Read the model definition and answer for the solid it produces. Units are mm, in the model's axes. A direction names the side the tool comes from. Coordinates: 2 decimals unless noted, no trailing zeros. Write each loop counter-clockwise with the first axis right and the second up, starting at its lowest first coordinate (ties: lowest second). Pieces come first, ordered by that corner, then holes.
from build123d import *

# Parameters (mm, degrees)
ESQUISSE1_R             = 20
BOSS_EXTRU_1_DEPTH      = 2
ESQUISSE2_R             = 3.025
BOSS_EXTRU_2_DEPTH      = 4
ESQUISSE4_R             = 10
BOSS_EXTRU_3_DEPTH      = 0.5
ENL_V_MAT_EXTRU_1_DEPTH = 6
ESQUISSE5_R             = 4.025
BOSS_EXTRU_4_DEPTH      = 1


with BuildPart() as part:
    # Esquisse1 → Boss.-Extru.1 (new body)
    with BuildSketch(Plane(origin=(0, 0, 0), x_dir=(1, 0, 0), z_dir=(0, 1, 0))):
        Circle(ESQUISSE1_R)
    extrude(amount=BOSS_EXTRU_1_DEPTH)

    # Esquisse2 → Boss.-Extru.2 (add)
    with BuildSketch(Plane(origin=(0, 2, 0), x_dir=(1, 0, 0), z_dir=(0, 1, 0))):
        with Locations((0, 16)):
            Circle(ESQUISSE2_R)
        with Locations((16, 0)):
            Circle(ESQUISSE2_R)
        with Locations((0, -16)):
            Circle(ESQUISSE2_R)
        with Locations((-16, 0)):
            Circle(ESQUISSE2_R)
    extrude(amount=BOSS_EXTRU_2_DEPTH)

    # Esquisse4 → Boss.-Extru.3 (add)
    with BuildSketch(Plane(origin=(0, 2, 0), x_dir=(1, 0, 0), z_dir=(0, 1, 0))):
        Circle(ESQUISSE4_R)
    extrude(amount=BOSS_EXTRU_3_DEPTH)

    # Esquisse3 → Enlèv. mat.-Extru.1 (cut)
    with BuildSketch(Plane(origin=(0, 2.5, 0), x_dir=(1, 0, 0), z_dir=(0, 1, 0))):
        Polygon((4.5, -7.794228634), (9, 0), (4.5, 7.794228634), (-4.5, 7.794228634), (-9, 0), (-4.5, -7.794228634), align=None)
    extrude(amount=-ENL_V_MAT_EXTRU_1_DEPTH, mode=Mode.SUBTRACT)

    # Esquisse5 → Boss.-Extru.4 (add)
    with BuildSketch(Plane(origin=(0, 2, 0), x_dir=(1, 0, 0), z_dir=(0, 1, 0))):
        with Locations((16, 0)):
            Circle(ESQUISSE5_R)
        with Locations((0, 16)):
            Circle(ESQUISSE5_R)
        with Locations((0, -16)):
            Circle(ESQUISSE5_R)
        with Locations((-16, 0)):
            Circle(ESQUISSE5_R)
    extrude(amount=BOSS_EXTRU_4_DEPTH)


solid = part.part
Item 1: The part is cut by section B-B (z = 6). Give the vertices of the cut face in (x, y).
Item 2: For faces 1 (the flat face through (-6.781, 1.268, 3.843)), 2 (the cylindrical face through (2.164, 2.493, -19.394)), 3 (the flat face through (16, 6, 0)), determine the directions among +Z, -Z, +X, -X, +Y, -Y from which every point of the face is accessible in a straight line to the end or side of a thin tool.
Item 3: Given pin 1 (1 mm diameter, centred on y = 3.5, z = 8, fed in from +X); pin 2 (3 mm diameter, centred on y = 3, z = 14.5, fed in from -X); pin 3 (1.5 mm diameter, centred on x = 8.5, y = 2, fed in from +Z); pin 4 (16 mm diameter, centred on x = 1, z = 1.5, fed in from +Y), each flat-ended and moving along its own axis, determine where each tip first touches the part or whether it passes through.
Item 4: Find the intervals of material crossed by probe 1 along Z at (x, y) = (0, 3.2) (3 decimals); probe 2 along Y at (x, z) = (-5.5, -6.5); probe 3 along X at (y, z) = (0.45, 0), in increasing order.
Item 5: The part is cut by section D-D (z = 16). Give the vertices of the cut face in (x, y) (3 decimals), and give its area (3 significant figures).
Item 6: The part is cut by section A-A (x = 0). Give the vertices of the cut face in (y, z) (3 decimals), and give its area (3 significant figures).
Item 7: The part is cut by section C-C (x = -16). Give the vertices of the cut face in (y, z) (3 decimals), and give its area (3 significant figures).
Answer:
1. outline: (-19.08, 0) - (-5.54, 0) - (-5.54, 2.5) - (-8, 2.5) - (-8, 2) - (-19.08, 2) - close; (5.54, 0) - (19.08, 0) - (19.08, 2) - (8, 2) - (8, 2.5) - (5.54, 2.5) - close
2. face 1: +Y, -Y
2. face 2: +Y
2. face 3: +Z, -Z, +X, -X, +Y
3. pin 1: passes through
3. pin 2: stops at x = -14.86
3. pin 3: stops at z = 18.44
3. pin 4: stops at y = 2.5
4. probe 1: z = -19.025 to -12.975, 12.975 to 19.025
4. probe 2: y = 0 to 2.5
4. probe 3: x = -20 to -9, 9 to 20
5. outline: (-12, 0) - (12, 0) - (12, 2) - (4.025, 2) - (4.025, 3) - (3.025, 3) - (3.025, 6) - (-3.025, 6) - (-3.025, 3) - (-4.025, 3) - (-4.025, 2) - (-12, 2) - close
5. area: 74.2 mm2
6. outline: (0, -20) - (2, -20) - (2, -20.025) - (3, -20.025) - (3, -19.025) - (6, -19.025) - (6, -12.975) - (3, -12.975) - (3, -11.975) - (2, -11.975) - (2, -10) - (2.5, -10) - (2.5, -7.794) - (0, -7.794) - close; (0, 7.794) - (2.5, 7.794) - (2.5, 10) - (2, 10) - (2, 11.975) - (3, 11.975) - (3, 12.975) - (6, 12.975) - (6, 19.025) - (3, 19.025) - (3, 20.025) - (2, 20.025) - (2, 20) - (0, 20) - close
6. area: 103 mm2
7. outline: (0, -12) - (2, -12) - (2, -4.025) - (3, -4.025) - (3, -3.025) - (6, -3.025) - (6, 3.025) - (3, 3.025) - (3, 4.025) - (2, 4.025) - (2, 12) - (0, 12) - close
7. area: 74.2 mm2
